Can you work these out from the drawing? Everything is in mm from the part's minimum corner. Coordinates: 2 decimals unless noted, no trailing zeros. Write each loop counter-clockwise with the first axis right and the second up, starting at its lowest first coordinate (ties: lowest second). Pieces come first, ordered by that corner, then holes. Notation, with made-up numbers: (-31, 35) -> (-10, 35) arc R22 cw to (-10, 59) -> close; hole circle Ø5 at (12, 6). An arc over 180 degrees is marked (long way). Use a Markdown table: item, result. Add a question column.
Item 1: Imagine slicing it at C-C, the plane y = 3.8. Count the separate pieces of the cut face and the enclosed holes in it, and give its area (3 significant figures).
Item 2: Imagine slicing it at A-A, the plane z = 60. Write out the boundary of the cut face in (x, y).
Item 3: If I drill on line 1 along X through (y, z) = (4.15, 67); line 2 along X through (y, z) = (3.65, 60); line 3 along Z through (x, y) = (66.75, 3.4), over which ranges is the centre line in solid material (lowest first)? Write a range as from..to.
Item 4: Will these pins go through, and if not, where does the flat tip stop? pin 1 Ø1.8 at (x, z) = (10, 53.25) entering from -Y; pin 2 Ø3 at (x, z) = (66.75, 110) entering from -Y; pin 3 Ø3 at (x, y) = (77.5, 3) entering from +Z; pin 4 Ø1.5 at (x, y) = (43, 1.5) entering from -Z.
Item 5: Imagine slicing it at D-D, the plane z = 77. Write out the boundary of the cut face in (x, y), and give its area (3 significant figures).
Item 6: Imagine slicing it at B-B, the plane x = 60. Write out the boundary of the cut face in (y, z), and give its area (3 significant figures).
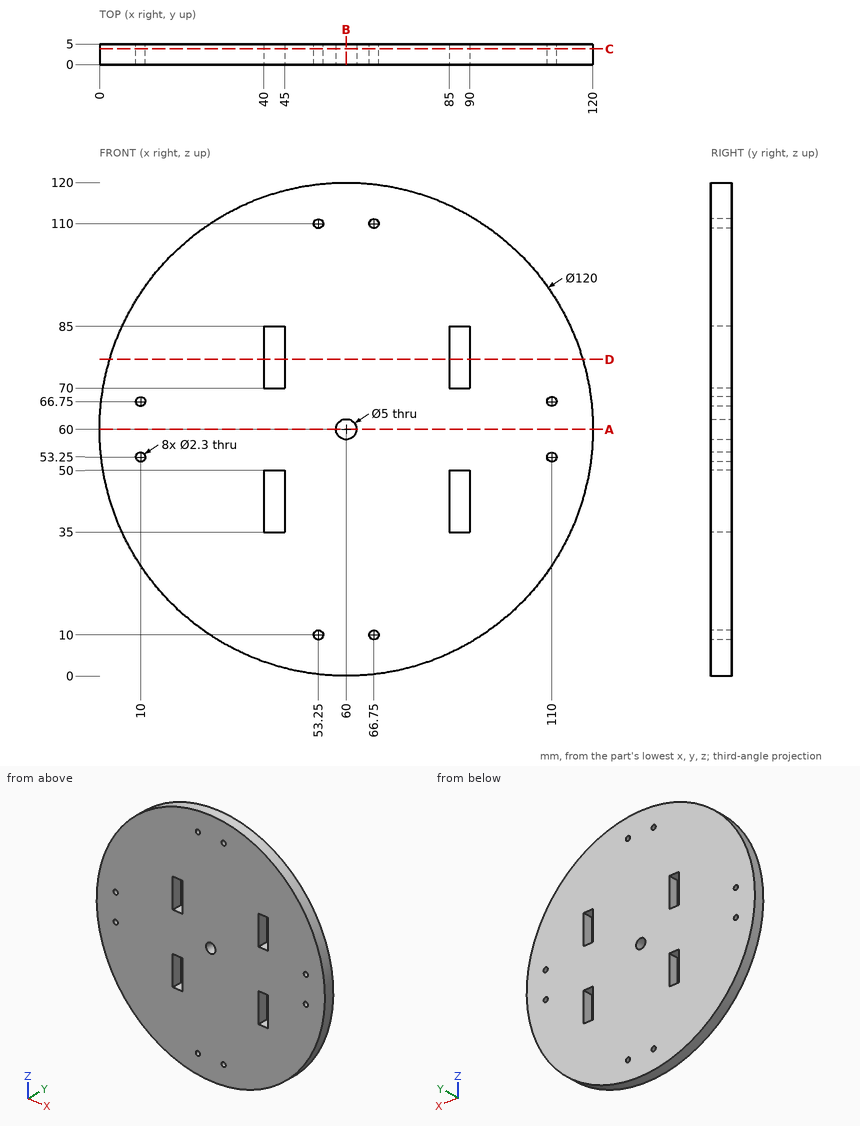
Ans:
| question | item | result |
|---|---|---|
| 1 | separate pieces | 1 |
| 1 | enclosed holes | 13 |
| 1 | area | 11,000 mm^2 |
| 2 | outline | (0, 0) -> (57.5, 0) -> (57.5, 5) -> (0, 5) -> close; (62.5, 0) -> (120, 0) -> (120, 5) -> (62.5, 5) -> close |
| 3 | line 1 | x = 0.41..8.88, 11.12..108.88, 111.12..119.59 |
| 3 | line 2 | x = 0..57.5, 62.5..120 |
| 3 | line 3 | z = 0.38..8.85, 11.15..108.85, 111.15..119.62 |
| 4 | pin 1 | passes through |
| 4 | pin 2 | stops at y = 0 |
| 4 | pin 3 | stops at z = 117.83 |
| 4 | pin 4 | stops at z = 2.24 |
| 5 | outline | (2.46, 0) -> (40, 0) -> (40, 5) -> (2.46, 5) -> close; (45, 0) -> (85, 0) -> (85, 5) -> (45, 5) -> close; (90, 0) -> (117.54, 0) -> (117.54, 5) -> (90, 5) -> close |
| 5 | area | 525 mm^2 |
| 6 | outline | (0, 0) -> (5, 0) -> (5, 57.5) -> (0, 57.5) -> close; (0, 62.5) -> (5, 62.5) -> (5, 120) -> (0, 120) -> close |
| 6 | area | 575 mm^2 |
